from build123d import *

# Parameters (mm, degrees)
CHAMFER1_SIZE     = 10
CIRPATTERN1_COUNT = 24
CHAMFER2_SIZE     = 1
CHAMFER3_SIZE     = 2


with BuildPart() as part:
    # Sketch1 → Revolve1 (revolve)
    with BuildSketch(Plane.XY, mode=Mode.PRIVATE) as revolve1_sk:
        Polygon((-187.5, 0), (-164.3, 0), (-164.3, 72), (-217, 72), (-217, 56), (-190, 56), (-190, 38), (-187.5, 38), align=None)
    revolve(revolve1_sk.sketch.rotate(Axis((0, 0, 0), (0, 1, 0)), 270), axis=Axis((0, 0, 0), (0, 1, 0)))

    # Chamfer1
    chamfer1_edges = [part.edges().sort_by_distance(p)[0] for p in [
        (0, 72, 164.3),
    ]]
    chamfer(chamfer1_edges, length=CHAMFER1_SIZE)

    # Sketch4 → M12x1.75 Tapped Hole1 (revolve, cut)
    with BuildSketch(Plane(origin=(0, 0, 174), x_dir=(0, 0, -1), z_dir=(1, 0, 0))):
        Polygon((0, 0), (0, 41.064389157), (5.1, 38), (5.1, 0), align=None)
    m12x1_75_tapped_hole1 = revolve(axis=Axis((0, -6.35, 174), (0, 1, 0)), mode=Mode.SUBTRACT)

    # CirPattern1: M12x1.75 Tapped Hole1 ×24 about axis
    cirpattern1_axis = Axis((0, 0, 0), (0, 1, 0))
    for i in range(1, CIRPATTERN1_COUNT):
        add(m12x1_75_tapped_hole1.rotate(cirpattern1_axis, i * 360 / CIRPATTERN1_COUNT), mode=Mode.SUBTRACT)

    # Chamfer2
    chamfer2_edges = [part.edges().sort_by_distance(p)[0] for p in [
        (0, 0, 187.5),
        (0, 38, 190),
        (0, 0, 164.3),
    ]]
    chamfer(chamfer2_edges, length=CHAMFER2_SIZE)

    # Chamfer3
    chamfer3_edges = [part.edges().sort_by_distance(p)[0] for p in [
        (0, 72, 217),
    ]]
    chamfer(chamfer3_edges, length=CHAMFER3_SIZE)


solid = part.part
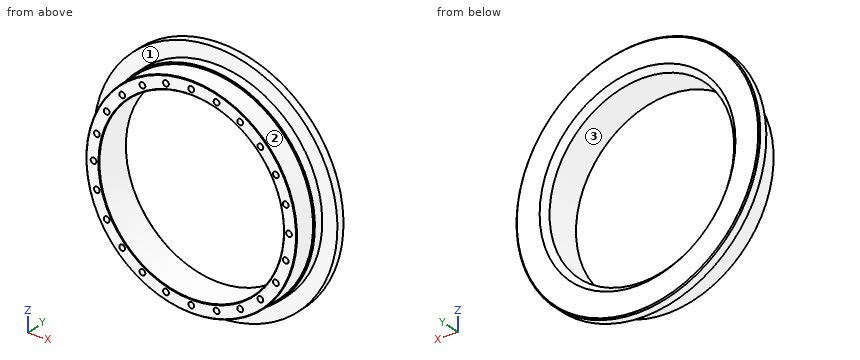
Geometry: final body of the model. Coordinates: model frame, mm. Face numbers are marked on the shaded views. Give positions to 0.01 mm unless a question says otherwise; leave off trailing zeros. Loops run counter-clockwise (first coordinate to the right, second up) from the corner with the lowest first, then second, coordinate; pieces in that order, holes last. Notation, with made-up numbers: (-20.5, 21) - (-2.5, 21) arc R13 cw to (-2.5, 25) - close; hole circle Ø1 at (11.25, 85). An arc over 180 degrees is marked (long way). Answer as CSV lines item,"result". Start each with the question number.
1. Draft query along Z for the marked faces 1, 2 and 3. Return one class per face: released by +Z, released by -Z, zero draft, split by the parting line, or undercut.
2. Section B-B, the plane y = 24. Give the number of separate pieces and of enclosed holes in the cut face, plus the area to 3 significant figures.
3. Ray query, L1, parallel to X at y = 16, z = 87; L2, parallel to X at y = 10, z = -49.5. Return the intervals inside material, ascending.
4. Section A-A, the plane y = 51. Return loops of the section in (x, z).
5. Pin query (flat end, axial travel): P1, Ø9, axis at x = 0, z = 174, coming from the -Y side; P2, Ø8, axis at x = 0, z = -174, coming from the -Y side; P3, Ø5, axis at y = 40.5, z = 129.5, coming from the -X side; P4, Ø2, axis at x = 140.5, z = 80.5, coming from the -Y side. Return the tip coordinate at first contact, or that it passes through.
Answers:
1,face 1,"zero draft"
1,face 2,"split by the parting line"
1,face 3,"undercut"
2,separate pieces,"1"
2,enclosed holes,"25"
2,area,"23,700 mm2"
3,L1,"x = -166.09 to -155.79, -145.59 to -139.38, 139.38 to 145.59, 155.79 to 166.09"
3,L2,"x = -180.85 to -170.53, -165.61 to -156.67, 156.67 to 165.61, 170.53 to 180.85"
4,outline,"circle Ø380 at (0, 0); hole circle Ø328.6 at (0, 0)"
5,P1,"stops at y = 38.36"
5,P2,"stops at y = 38.66"
5,P3,"stops at x = -141.32"
5,P4,"passes through"
